Autodesk Inventor part; units mm, degrees
ref_plane "YZ Plane" through (0, 0, 0) normal (1, 0, 0) x (0, 1, 0)
ref_plane "XZ Plane" through (0, 0, 0) normal (0, 1, 0) x (-1, 0, 0)
ref_plane "XY Plane" through (0, 0, 0) normal (0, 0, 1) x (1, 0, 0)
sketch "Sketch1" plane through (0, 0, 0) normal (0, 1, 0) x (-1, 0, 0)
  circle A0 centre (0, 0) radius 8
  dimension "d0" = 16
extrude "Extrusion1" add sketch "Sketch1" along normal blind 8
sketch "Sketch2" plane through (0, 8, 0) normal (0, 1, 0) x (1, 0, 0)
  circle A0 centre (0, 0) radius 8
  circle A1 centre (0, 0) radius 1.5
  dimension "d3" = 3
extrude "Extrusion2" add sketch "Sketch2" along normal blind 4.5 contours A1
sketch "Sketch3" plane through (0, 0, 0) normal (0, -1, 0) x (1, 0, 0)
  circle A0 centre (0, 0) radius 8
  circle A1 centre (0, 0) radius 7.5
  dimension "d6" = 15
extrude "Extrusion3" cut sketch "Sketch3" against normal blind 6.5 contours A1
sketch "Sketch4" plane through (0, 6.5, 0) normal (0, -1, 0) x (1, 0, 0)
  circle A0 centre (0, 0) radius 7.5
  circle A1 centre (0, 0) radius 7
  line L0 (0, 0) -> (7.5, 0)
  circle A2 centre (0, 0) radius 7.5
  line L1 (0, 0) -> (6.9038, -2.9305)
  point P0 (6.4435, -2.7351)
  point P1 (6.9038, -2.9305)
  point P2 (7, 0)
  dimension "d9" = 14
  dimension "d10" = 23
extrude "Extrusion4" add sketch "Sketch4" along normal blind 6.2 contours A0 L1 A1 L0 picked at (6.8601, -2.5496)
pattern_circular "Circular Pattern1" count 10 over 360 about axis through (0, 0, 0) along (0, 1, 0) of "Extrusion4"
sketch "Sketch5" plane through (0, 8, 0) normal (0, 1, 0) x (1, 0, 0)
  circle A0 centre (0, 0) radius 2.5
  circle A1 centre (0, 0) radius 6.5
  line L0 (-10, -1) -> (-10, 1)
  line L1 (-10, 1) -> (10, 1)
  line L2 (10, 1) -> (10, -1)
  line L3 (10, -1) -> (-10, -1)
  line L4 (-10, -1) -> (10, 1) construction
  line L5 (-10, 1) -> (10, -1) construction
  line L6 (0, 0) -> (3.25, 5.6292)
  line L7 (0, 0) -> (-6.5, 0)
  line L8 (-5.866, -8.1603) -> (-4.134, -9.1603)
  line L9 (-4.134, -9.1603) -> (5.866, 8.1603)
  line L10 (5.866, 8.1603) -> (4.134, 9.1603)
  line L11 (4.134, 9.1603) -> (-5.866, -8.1603)
  line L12 (-5.866, -8.1603) -> (5.866, 8.1603) construction
  line L13 (-4.134, -9.1603) -> (4.134, 9.1603) construction
  point P0 (0.2796, 2.4843)
  point P1 (2.3453, 6.0621)
  point P2 (-6.4226, 1)
  point P3 (-2.2913, 1)
  dimension "d16" = 5
  dimension "d17" = 13
  dimension "d18" = 2
  dimension "d19" = 20
  dimension "d20" = 120
  dimension "d21" = 2
  dimension "d22" = 20
extrude "Extrusion5" cut sketch "Sketch5" against normal blind 6.2 contours A0 L1 A1 L11
pattern_circular "Circular Pattern2" count 3 over 360 about axis through (0, 8, 0) along (0, -1, 0) of "Extrusion5"
fillet "Fillet1" radius 1.5 2 edges at (-6.4226, 7.25, -1) (2.3453, 7.25, -6.0621)
pattern_circular "Circular Pattern3" count 3 over 360 about axis through (0, 8, 0) along (0, 1, 0) of "Fillet1"
fillet "Fillet2" radius 1 2 edges at (-2.2913, 7.25, -1) (0.2796, 7.25, -2.4843)
pattern_circular "Circular Pattern4" count 3 over 360 about axis through (0, 8, 0) along (0, 1, 0) of "Fillet2"
chamfer "Chamfer1" distance 0.8 angle 30 1 edges at (8, 8, 0) measured on face at (-6.1962, 8, 0)
sketch "Sketch6" plane through (0, 6.5, 0) normal (0, -1, 0) x (1, 0, 0)
  arc A0 (0, 6.5) -> (-5.6292, 3.25) centre (0, 0) ccw
  arc A1 (1.299, 4.25) -> (0, 6.5) centre (0, 5) ccw
  line L0 (1.299, 4.25) -> (0.5701, 2.9875)
  arc A2 (-0.2114, 2.491) -> (0.5701, 2.9875) centre (-0.2959, 3.4875) ccw
  arc A3 (-0.2114, 2.491) -> (-2.0516, 1.4286) centre (0, 0) ccw
  arc A4 (-2.8723, 1) -> (-2.0516, 1.4286) centre (-2.8723, 2) ccw
  line L1 (-2.8723, 1) -> (-4.3301, 1)
  arc A5 (-5.6292, 3.25) -> (-4.3301, 1) centre (-4.3301, 2.5) ccw
  arc A6 (5.6292, -3.25) -> (5.6292, 3.25) centre (0, 0) ccw
  arc A7 (3.0311, -3.25) -> (5.6292, -3.25) centre (4.3301, -2.5) ccw
  line L2 (3.0311, -3.25) -> (2.3022, -1.9875)
  arc A8 (2.263, -1.0625) -> (2.3022, -1.9875) centre (3.1682, -1.4875) ccw
  arc A9 (2.263, -1.0625) -> (2.263, 1.0625) centre (0, 0) ccw
  arc A10 (2.3022, 1.9875) -> (2.263, 1.0625) centre (3.1682, 1.4875) ccw
  line L3 (2.3022, 1.9875) -> (3.0311, 3.25)
  arc A11 (5.6292, 3.25) -> (3.0311, 3.25) centre (4.3301, 2.5) ccw
  arc A12 (-5.6292, -3.25) -> (0, -6.5) centre (0, 0) ccw
  arc A13 (-4.3301, -1) -> (-5.6292, -3.25) centre (-4.3301, -2.5) ccw
  line L4 (-4.3301, -1) -> (-2.8723, -1)
  arc A14 (-2.0516, -1.4286) -> (-2.8723, -1) centre (-2.8723, -2) ccw
  arc A15 (-2.0516, -1.4286) -> (-0.2114, -2.491) centre (0, 0) ccw
  arc A16 (0.5701, -2.9875) -> (-0.2114, -2.491) centre (-0.2959, -3.4875) ccw
  line L5 (0.5701, -2.9875) -> (1.299, -4.25)
  arc A17 (0, -6.5) -> (1.299, -4.25) centre (0, -5) ccw
  line L6 (7.3078, 1.6871) -> (6.8206, 1.5747)
  arc A18 (6.8206, 1.5747) -> (5.6631, 4.1145) centre (0, 0) ccw
  line L7 (5.6631, 4.1145) -> (6.0676, 4.4084)
  arc A19 (6.0676, 4.4084) -> (4.9204, 5.6603) centre (0, 0) ccw
  line L8 (4.9204, 5.6603) -> (4.5924, 5.283)
  arc A20 (4.5924, 5.283) -> (2.1631, 6.6574) centre (0, 0) ccw
  line L9 (2.1631, 6.6574) -> (2.3176, 7.1329)
  arc A21 (2.3176, 7.1329) -> (0.6537, 7.4715) centre (0, 0) ccw
  line L10 (0.6537, 7.4715) -> (0.6101, 6.9734)
  arc A22 (0.6101, 6.9734) -> (-2.1631, 6.6574) centre (0, 0) ccw
  line L11 (-2.1631, 6.6574) -> (-2.3176, 7.1329)
  arc A23 (-2.3176, 7.1329) -> (-3.8628, 6.4288) centre (0, 0) ccw
  line L12 (-3.8628, 6.4288) -> (-3.6053, 6.0002)
  arc A24 (-3.6053, 6.0002) -> (-5.6631, 4.1145) centre (0, 0) ccw
  line L13 (-5.6631, 4.1145) -> (-6.0676, 4.4084)
  arc A25 (-6.0676, 4.4084) -> (-6.9038, 2.9305) centre (0, 0) ccw
  line L14 (-6.9038, 2.9305) -> (-6.4435, 2.7351)
  arc A26 (-6.4435, 2.7351) -> (-7, 0) centre (0, 0) ccw
  line L15 (-7, 0) -> (-7.5, 0)
  arc A27 (-7.5, 0) -> (-7.3078, -1.6871) centre (0, 0) ccw
  line L16 (-7.3078, -1.6871) -> (-6.8206, -1.5747)
  arc A28 (-6.8206, -1.5747) -> (-5.6631, -4.1145) centre (0, 0) ccw
  line L17 (-5.6631, -4.1145) -> (-6.0676, -4.4084)
  arc A29 (-6.0676, -4.4084) -> (-4.9204, -5.6603) centre (0, 0) ccw
  line L18 (-4.9204, -5.6603) -> (-4.5924, -5.283)
  arc A30 (-4.5924, -5.283) -> (-2.1631, -6.6574) centre (0, 0) ccw
  line L19 (-2.1631, -6.6574) -> (-2.3176, -7.1329)
  arc A31 (-2.3176, -7.1329) -> (-0.6537, -7.4715) centre (0, 0) ccw
  line L20 (-0.6537, -7.4715) -> (-0.6101, -6.9734)
  arc A32 (-0.6101, -6.9734) -> (2.1631, -6.6574) centre (0, 0) ccw
  line L21 (2.1631, -6.6574) -> (2.3176, -7.1329)
  arc A33 (2.3176, -7.1329) -> (3.8628, -6.4288) centre (0, 0) ccw
  line L22 (3.8628, -6.4288) -> (3.6053, -6.0002)
  arc A34 (3.6053, -6.0002) -> (5.6631, -4.1145) centre (0, 0) ccw
  line L23 (5.6631, -4.1145) -> (6.0676, -4.4084)
  arc A35 (6.0676, -4.4084) -> (6.9038, -2.9305) centre (0, 0) ccw
  line L24 (6.9038, -2.9305) -> (6.4435, -2.7351)
  arc A36 (6.4435, -2.7351) -> (7, 0) centre (0, 0) ccw
  line L25 (7, 0) -> (7.5, 0)
  arc A37 (7.5, 0) -> (7.3078, 1.6871) centre (0, 0) ccw
  circle A38 centre (0, 0) radius 1.5
  dimension "d39" = 3
extrude "Extrusion6" add sketch "Sketch6" along normal blind 5 contours A38
sketch "Sketch7" plane through (0, 8, 0) normal (0, 1, 0) x (1, 0, 0)
  circle A0 centre (0, 0) radius 1.5
  arc A1 (0, 6.5) -> (-5.6292, 3.25) centre (0, 0) ccw
  arc A2 (1.299, 4.25) -> (0, 6.5) centre (0, 5) ccw
  line L0 (1.299, 4.25) -> (0.5701, 2.9875)
  arc A3 (-0.2114, 2.491) -> (0.5701, 2.9875) centre (-0.2959, 3.4875) ccw
  arc A4 (-0.2114, 2.491) -> (-2.0516, 1.4286) centre (0, 0) ccw
  arc A5 (-2.8723, 1) -> (-2.0516, 1.4286) centre (-2.8723, 2) ccw
  line L1 (-2.8723, 1) -> (-4.3301, 1)
  arc A6 (-5.6292, 3.25) -> (-4.3301, 1) centre (-4.3301, 2.5) ccw
  arc A7 (5.6292, -3.25) -> (5.6292, 3.25) centre (0, 0) ccw
  arc A8 (3.0311, -3.25) -> (5.6292, -3.25) centre (4.3301, -2.5) ccw
  line L2 (3.0311, -3.25) -> (2.3022, -1.9875)
  arc A9 (2.263, -1.0625) -> (2.3022, -1.9875) centre (3.1682, -1.4875) ccw
  arc A10 (2.263, -1.0625) -> (2.263, 1.0625) centre (0, 0) ccw
  arc A11 (2.3022, 1.9875) -> (2.263, 1.0625) centre (3.1682, 1.4875) ccw
  line L3 (2.3022, 1.9875) -> (3.0311, 3.25)
  arc A12 (5.6292, 3.25) -> (3.0311, 3.25) centre (4.3301, 2.5) ccw
  arc A13 (-5.6292, -3.25) -> (0, -6.5) centre (0, 0) ccw
  arc A14 (-4.3301, -1) -> (-5.6292, -3.25) centre (-4.3301, -2.5) ccw
  line L4 (-4.3301, -1) -> (-2.8723, -1)
  arc A15 (-2.0516, -1.4286) -> (-2.8723, -1) centre (-2.8723, -2) ccw
  arc A16 (-2.0516, -1.4286) -> (-0.2114, -2.491) centre (0, 0) ccw
  arc A17 (0.5701, -2.9875) -> (-0.2114, -2.491) centre (-0.2959, -3.4875) ccw
  line L5 (0.5701, -2.9875) -> (1.299, -4.25)
  arc A18 (0, -6.5) -> (1.299, -4.25) centre (0, -5) ccw
  circle A19 centre (0, 0) radius 7.2
  line L6 (0, 0) -> (-6, 0)
  circle A20 centre (-6, 0) radius 0.75
  dimension "d42" = 6
  dimension "d43" = 1.5
extrude "Extrusion7" cut sketch "Sketch7" against normal blind 5 contours A20
pattern_circular "Circular Pattern5" count 3 over 360 about axis through (0, 8, 0) along (0, 1, 0) of "Extrusion7"
properties part number "motor_1608_outer"
Check sheet for the modelled part. Datum: model origin and axes. Units: mm. A direction names the side the tool comes from. Round coordinates to 2 decimals unless told otherwise and drop trailing zeros. Loops run counter-clockwise (first coordinate to the right, second up) from the corner with the lowest first, then second, coordinate; pieces in that order, holes last. Notation, with made-up numbers: M -34,17.5 L -10,17.5 A27 cw -10,41.5 Z; hole C 42.5,59.25 d7. An arc over 180 degrees is marked long. One line per item, written item: value.
(1) Depth check by flat-ended pin: pin 1 Ø3.5 at (x, z) = (0, 0.5) entering from -Y; pin 2 Ø3 at (x, y) = (-3, 4.5) entering from +Z; pin 3 Ø2.5 at (x, z) = (-6, 0) entering from +Y. Enter the tip coordinate at first touch or a pass-through.
Computed values:
pin 1: stops at y = 1.5
pin 2: stops at z = 7.86
pin 3: stops at y = 8
(2) Sectioned sample at B-B, the plane y = 10. Record the cut outline in (x, z).
Computed values:
outline: C 0,0 d3
(3) Thickness scan on line 1 (Z direction, x = 0, y = 5.5); line 2 (X direction, y = 2, z = -1); line 3 (Z direction, x = 3, y = 7.35). Record the ranges inside material, lowest first.
Computed values:
line 1: z = -8 to -7, -1.5 to 1.5, 7 to 8
line 2: x = -7.94 to -7.43, -1.12 to 1.12, 6.93 to 7.94
line 3: z = -7.42 to -5.95, -4.45 to -3.2, 3.2 to 4.45, 5.95 to 7.42
(4) Access from +Z, -Z, +X, -X, +Y, -Y to the whole of each face (thin tool, end or side, straight path). Record for faces 1 (the face through (-6.6, 0.3, -3)), 2 (the face through (-1.26, 7.26, 2.16)).
Computed values:
face 1: -Y
face 2: +Y, -Y
(5) Sectioned sample at A-A, the plane y = 3.75. Count the separate pieces of the cut face and the enclosed holes in it, then the cut area to 3 significant figures.
Computed values:
separate pieces: 2
enclosed holes: 1
area: 46.0 mm^2
